```python
from build123d import *

# Parameters (mm, degrees)
F1_DEPTH = 3


with BuildPart() as f1:
    # F0 (on Front) → F1 (new body)
    with BuildSketch(Plane.XZ):
        with BuildLine():
            Line((0, 110), (0, -110))
            ThreePointArc((0, -110), (56.599092, -94.321486), (97.063827, -51.755323))
            Line((97.063827, -51.755323), (121.953153, -41.987608))
            Line((121.953153, -41.987608), (109.51686, -10.298421))
            ThreePointArc((109.51686, -10.298421), (109.801283, 6.608946), (107.490949, 23.360135))
            Line((107.490949, 23.360135), (80.694538, 33.874987))
            Line((80.694538, 33.874987), (91.411813, 61.187258))
            ThreePointArc((91.411813, 61.187258), (51.814099, 97.032465), (0, 110))
        make_face()
    extrude(amount=F1_DEPTH)


solid = f1.part
```
For this review, take the finished solid that the model builds, in its own axes (mm). A direction names the side the tool comes from. Give positions to 0.01 mm unless a question says otherwise; leave off trailing zeros. Write each loop counter-clockwise with the first axis right and the second up, starting at its lowest first coordinate (ties: lowest second). Pieces come first, ordered by that corner, then holes. Notation, with made-up numbers: M 10.25,14 L 49.25,14 A24 ccw 49.25,32 Z; hole C 9.25,73 d3. An arc over 180 degrees is marked long. Answer as a JSON object with one key per item and string values. Group by question number.
Item 1: For pin 1 Ø1.5 at (y, z) = (-2, -7) entering from +X, flat-tipped, find the tip position at first contact; note if it passes through.
Item 2: Draft analysis for pull direction Z (two halves, no side actions). For faces 1 (the flat face through (94.28, -1.479, 28.544)), 2 (the cylindrical face through (52.479, -1.479, 96.674)), 3 (the flat face through (47, 0, 2)), state which applies: +Z half, -Z half, draft (parallel to the pull), parting line (faces both ways), or undercut.
Item 3: Consider section C-C on x = 23. Write out the cut boundary in (y, z), plus the area to 3 significant figures.
Item 4: For probe 1 along Z at (x, y) = (66.5, -2.2); probe 2 along Z at (x, y) = (19, -1.85); probe 3 along X at (y, z) = (-0.6, -34.5), list the stretches that pass through material, from the lowest coordinate up. Write a range as [from, to].
Item 5: Consider section B-B on z = 88. Write out the cut boundary in (x, y).
Item 6: Consider section A-A on y = -1.35. Write out the cut boundary in (x, z), plus the area to 3 significant figures.
Item 7: Tool access review of faces 4 (the flat face through (85.98, -1.48, 47.34)), 5 (the flat face through (47, -3, 2)): name each direction out of +Z, -Z, +X, -X, +Y, -Y from which nothing blocks a thin tool from reaching the whole face with its end or side.
Check result:
{
 "1": {"pin 1": "stops at x = 109.82"},
 "2": {"face 1": "undercut", "face 2": "+Z half", "face 3": "draft"},
 "3": {"outline": "M -3,-107.57 L 0,-107.57 L 0,107.57 L -3,107.57 Z", "area": "645 mm^2"},
 "4": {"probe 1": "z = [-87.62, 87.62]", "probe 2": "z = [-108.35, 108.35]", "probe 3": "x = [0, 119.01]"},
 "5": {"outline": "M 0,-3 L 66,-3 L 66,0 L 0,0 Z"},
 "6": {"outline": "M 0,-110 A110 ccw 97.06,-51.76 L 121.95,-41.99 L 109.52,-10.3 A110 ccw 107.49,23.36 L 80.69,33.87 L 91.41,61.19 A110 ccw 0,110 Z", "area": "18,900 mm^2"},
 "7": {"face 4": "+X, +Y, -Y", "face 5": "+Z, -Z, +X, -X, -Y"}
}
